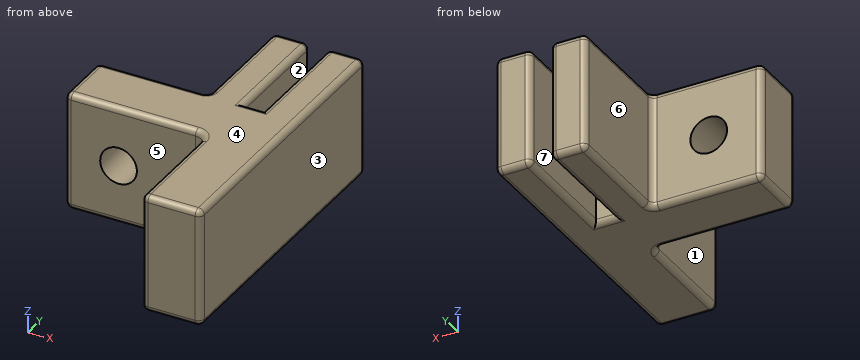
```python
from build123d import *

# Parameters (mm, degrees)
SKETCH1_W           = 3
SKETCH1_H           = 10
BOSS_EXTRUDE1_DEPTH = 10
SKETCH3_R           = 1.55
CUT_EXTRUDE1_DEPTH  = 10
FILLET1_R           = 1
FILLET2_R           = 0.5


with BuildPart() as part:
    # Sketch1 → Boss-Extrude1 (new body)
    with BuildSketch(Plane.XY):
        Polygon((6, -5), (6, 5), (-6, 5), (-6, 10), (11, 10), (11, -5), align=None)
        with Locations((4.85, 15)):
            Rectangle(SKETCH1_W, SKETCH1_H)
        with Locations((9.5, 15)):
            Rectangle(SKETCH1_W, SKETCH1_H)
    extrude(amount=BOSS_EXTRUDE1_DEPTH)

    # Sketch3 → Cut-Extrude1 (cut)
    with BuildSketch(Plane.XZ.offset(-5)):
        with Locations(Location((-1.5, 5, 0), (0, 0, 270))):
            Circle(SKETCH3_R)
    extrude(amount=-CUT_EXTRUDE1_DEPTH, mode=Mode.SUBTRACT)

    # Fillet1
    fillet1_edges = [part.edges().sort_by_distance(p)[0] for p in [
        (6, 5, 5),
    ]]
    fillet(fillet1_edges, radius=FILLET1_R)

    # Fillet2
    fillet2_edges = [part.edges().sort_by_distance(p)[0] for p in [
        (8.5, -5, 10),
        (-0.5, 5, 0),
        (-6, 7.5, 0),
        (11, 7.5, 10),
        (-1.325, 10, 0),
        (3.35, 15, 0),
        (4.85, 20, 0),
        (6.35, 15, 0),
        (7.175, 10, 0),
        (8, 15, 0),
        (9.5, 20, 0),
        (11, 7.5, 0),
        (8.5, -5, 0),
        (6, -0.5, 0),
        (9.5, 20, 10),
        (-6, 5, 5),
        (-6, 10, 5),
        (3.35, 10, 5),
        (3.35, 20, 5),
        (6.35, 20, 5),
        (8, 20, 5),
        (11, 20, 5),
        (11, -5, 5),
        (6, -5, 5),
        (8, 15, 10),
        (7.175, 10, 10),
        (6.35, 15, 10),
        (4.85, 20, 10),
        (5.707106781, 4.707106781, 0),
        (5.707106781, 4.707106781, 10),
        (3.35, 15, 10),
        (6, -0.5, 10),
        (-1.325, 10, 10),
        (-6, 7.5, 10),
        (-0.5, 5, 10),
    ]]
    fillet(fillet2_edges, radius=FILLET2_R)


solid = part.part
```
Can you work these out from the model? Positions are in its coordinate system, mm. Face numbers are marked on the shaded views. A direction names the side the tool comes from. Round coordinates to 2 decimals unless told otherwise and drop trailing zeros. Loops run counter-clockwise (first coordinate to the right, second up) from the corner with the lowest first, then second, coordinate; pieces in that order, holes last.
Item 1: Will these pins go through, and if not, where does the flat tip stop? pin 1 Ø4 at (x, z) = (-1.5, 5) entering from -Y; pin 2 Ø2.5 at (y, z) = (15, 4) entering from -X; pin 3 Ø1.8 at (x, z) = (7, 7) entering from +Y.
Item 2: If we mould it in two halves opening along X, with no side actions, what happens to the marked faces 1, 2, 3 and 4? For each: +X half, -X half, draft (parallel to the pull), parting line (faces both ways), or undercut.
Item 3: Suppose I cut it at B-B, the plane x = -1.5. Write out the boundary of the cut face in (y, z).
Item 4: Please list where these lines run through material, in increasing order: L1, parallel to X at y = 7, z = 5; L2, parallel to X at y = 10.5, z = 2; L3, parallel to X at y = 2, z = 8.25.
Item 5: Suppose I cut it at A-A, the plane z = 5. Write out the boundary of the cut face in (x, y), then the cut area to 3 significant figures.
Item 6: Suppose I cut it at C-C, the plane y = 14.25. Write out the boundary of the cut face in (x, z), then the cut area to 3 significant figures.
Item 7: Suppose I cut it at D-D, the plane x = -3.75. Write out the boundary of the cut face in (y, z), then the cut area to 3 significant figures.
Item 8: Which directions (+Z, -Z, +X, -X, +Y, -Y) give clear straight access to the entire face, cutting with the end or side of a thin tool? Please do the marked faces 5, 6 and 7.
Reported:
1. pin 1: stops at y = 5
1. pin 2: stops at x = 3.35
1. pin 3: stops at y = 19.93
2. face 1: -X half
2. face 2: undercut
2. face 3: +X half
2. face 4: draft
3. outline: (5, 0.5) arc R0.5 ccw to (5.5, 0) - (9.5, 0) arc R0.5 ccw to (10, 0.5) - (10, 3.45) - (5, 3.45) - close; (5, 6.55) - (10, 6.55) - (10, 9.5) arc R0.5 ccw to (9.5, 10) - (5.5, 10) arc R0.5 ccw to (5, 9.5) - close
4. L1: x = -6 to -3.05, 0.05 to 11
4. L2: x = 3.35 to 6.35, 8 to 11
4. L3: x = 6 to 11
5. outline: (-6, 5.5) arc R0.5 ccw to (-5.5, 5) - (-3.05, 5) - (-3.05, 10) - (-5.5, 10) arc R0.5 ccw to (-6, 9.5) - close; (0.05, 5) - (5, 5) arc R1 cw to (6, 4) - (6, -4.5) arc R0.5 ccw to (6.5, -5) - (10.5, -5) arc R0.5 ccw to (11, -4.5) - (11, 19.5) arc R0.5 ccw to (10.5, 20) - (8.5, 20) arc R0.5 ccw to (8, 19.5) - (8, 10) - (6.35, 10) - (6.35, 19.5) arc R0.5 ccw to (5.85, 20) - (3.85, 20) arc R0.5 ccw to (3.35, 19.5) - (3.35, 10.5) arc R0.5 cw to (2.85, 10) - (0.05, 10) - close
5. area: 179 mm2
6. outline: (3.35, 0.5) arc R0.5 ccw to (3.85, 0) - (5.85, 0) arc R0.5 ccw to (6.35, 0.5) - (6.35, 9.5) arc R0.5 ccw to (5.85, 10) - (3.85, 10) arc R0.5 ccw to (3.35, 9.5) - close; (8, 0.5) arc R0.5 ccw to (8.5, 0) - (10.5, 0) arc R0.5 ccw to (11, 0.5) - (11, 9.5) arc R0.5 ccw to (10.5, 10) - (8.5, 10) arc R0.5 ccw to (8, 9.5) - close
6. area: 59.6 mm2
7. outline: (5, 0.5) arc R0.5 ccw to (5.5, 0) - (9.5, 0) arc R0.5 ccw to (10, 0.5) - (10, 9.5) arc R0.5 ccw to (9.5, 10) - (5.5, 10) arc R0.5 ccw to (5, 9.5) - close
7. area: 49.8 mm2
8. face 5: +Z, -Z, -X, -Y
8. face 6: +Z, -Z, -X, +Y
8. face 7: +Z, -Z, +Y
